Geometry: final body of the model. Coordinates: model frame, mm. A direction names the side the tool comes from. Round coordinates to 2 decimals unless told otherwise and drop trailing zeros. Loops run counter-clockwise (first coordinate to the right, second up) from the corner with the lowest first, then second, coordinate; pieces in that order, holes last. Notation, with made-up numbers: M -27,53.5 L -6,53.5 A19 cw -6,68.5 Z; hole C 38,51.5 d4. An arc over 180 degrees is marked long. Return JSON: item names as keys, results as strings.
Autodesk Inventor part; units mm, degrees
ref_plane "Start plane" through (0, 0, 0) normal (0, 0, 1) x (1, 0, 0)
ref_plane "End plane" through (0, 0, 2200) normal (0, 0, 1) x (1, 0, 0)
ref_plane "YZ Plane" through (0, 0, 0) normal (1, 0, 0) x (0, 1, 0)
ref_plane "Start plane" through (0, 0, 0) normal (0, 0, 1) x (1, 0, 0)
ref_plane "End plane" through (0, 0, 2200) normal (0, 0, 1) x (1, 0, 0)
sketch "Sketch" plane through (0, 0, 0) normal (0, 0, 1) x (1, 0, 0)
  line L0 (-1.51, 0) -> (-1.51, 50)
  line L1 (-1.51, 50) -> (48.49, 50)
  line L2 (48.49, 50) -> (48.49, 48.3694)
  line L3 (44.4604, 43.894) -> (11.5538, 40.4354)
  line L4 (4.39, 32.4792) -> (4.39, 0)
  line L5 (4.39, 0) -> (-1.51, 0) construction
  line L6 (26.44, 50) -> (26.44, 42) construction
  line L7 (48.49, 44.3175) -> (48.49, 42) construction
  line L8 (48.49, 42) -> (26.44, 42) construction
  line L9 (0, 15) -> (0, -27) construction
  line L10 (-5.539, 0) -> (16.0067, 0) construction
  line L11 (-1.51, 0) -> (-1.51, -50)
  line L12 (-1.51, -50) -> (48.49, -50)
  line L13 (48.49, -50) -> (48.49, -48.3694)
  line L14 (44.4604, -43.894) -> (11.5538, -40.4354)
  line L15 (4.39, -32.4792) -> (4.39, 0)
  arc A0 (11.5538, 40.4354) -> (4.39, 32.4792) centre (12.39, 32.4792) ccw
  arc A1 (4.39, -32.4792) -> (11.5538, -40.4354) centre (12.39, -32.4792) ccw
  arc A2 (44.4604, 43.894) -> (48.49, 48.3694) centre (43.99, 48.3694) ccw
  arc A3 (48.49, -48.3694) -> (44.4604, -43.894) centre (43.99, -48.3694) ccw
  line L16 (0, 70) -> (0, -70) construction
  line L17 (-16.5166, 0) -> (60.3266, 0) construction
  point P0 (4.39, 39.6825)
  point P1 (48.49, -44.3175)
  point P2 (4.39, -39.6825)
  point P3 (26.44, -50)
  point P4 (26.44, -42)
  dimension "d0" = 5.9
  dimension "d1" = 50
  dimension "d2" = 50
  dimension "d3" = 8
  dimension "d4" = 22.05
  dimension "d5" = 2.3175
  dimension "d23" = 8
  dimension "d24" = 4.5
  dimension "d25" = 1.51
extrude "Body" add sketch "Sketch" along normal up to surface (2200 mm away) from surface at 0
sketch "Sketch3" plane through (0, 0, 0) normal (0, 0, 1) x (1, 0, 0)
  line L0 (0, 0) -> (10, 0)
ref_plane "Work Plane3" through (0, 0, 0) normal (0, -1, 0) x (1, 0, 0)
sketch "Sketch4" plane through (0, 0, 0) normal (0, -1, 0) x (1, 0, 0)
  line L0 (-2, 0) -> (12, 0)
  line L1 (-2, 2200) -> (12, 2200)
  dimension "d29" = 2200
equation "\"d0\" = G_T"
equation "\"d1\" = 0.5 * G_H"
equation "\"d2\" = G_W"
equation "\"d3\" = G_T1"
equation "\"d4\" = G_C"
equation "\"d23\" = G_IR"
equation "\"d24\" = G_ER"
equation "\"d25\" = ex"
equation "\"d6\" = G_L"
equation "\"G_W\" = 50"
equation "\"G_T\" = 5.9"
equation "\"G_T1\" = 8"
equation "\"G_NG\" = 0.105104"
equation "\"G_ER\" = 4.5"
equation "\"G_IR\" = 8"
equation "\"G_C\" = 22.05"
equation "\"G_L\" = d29"
equation "\"ex\" = 1.51"
equation "\"G_OFFSET_START\" = 0"
equation "\"G_OFFSET_END\" = 0"
properties part number "ISO 657/11 - CH 100 x 10 - 2200" material "Steel, Mild"
Q1. Reachability of faces 1 (the flat face through (4.39, 0, 1085)), 2 (the flat face through (-1.51, 1, 1085)) from +Z, -Z, +X, -X, +Y, -Y: full face, straight path, thin tool, end or side. Return the list, or none.
Determined:
{"face 1": "+Z, -Z, +X", "face 2": "+Z, -Z, -X, +Y, -Y"}
Q2. Section query B-B (z = 761.5). Output: boundary loops of the cut face in (x, y), plus the area to 3 significant figures.
Determined:
{"outline": "M -1.51,-50 L 48.49,-50 L 48.49,-48.37 A4.5 ccw 44.46,-43.89 L 11.55,-40.44 A8 cw 4.39,-32.48 L 4.39,32.48 A8 cw 11.55,40.44 L 44.46,43.89 A4.5 ccw 48.49,48.37 L 48.49,50 L -1.51,50 Z", "area": "1,310 mm^2"}
Q3. Material intervals for L1, parallel to Y at x = 44, z = 702; L2, parallel to Y at x = 13.5, z = 538.5; L3, parallel to X at y = 33, z = 314.5, sorted ascending.
Determined:
{"L1": "y = -50 to -43.85, 43.85 to 50", "L2": "y = -50 to -40.64, 40.64 to 50", "L3": "x = -1.51 to 4.41"}
Q4. Section query C-C (y = -16). Output: boundary loops of the cut face in (x, z).
Determined:
{"outline": "M -1.51,0 L 4.39,0 L 4.39,2200 L -1.51,2200 Z"}
Q5. Section query A-A (x = 19.5). Output: boundary loops of the cut face in (y, z), plus the area to 3 significant figures.
Determined:
{"outline": "M -50,0 L -41.27,0 L -41.27,2200 L -50,2200 Z; M 41.27,0 L 50,0 L 50,2200 L 41.27,2200 Z", "area": "38,400 mm^2"}
Q6. Pin query (flat end, axial travel): pin 1 (4 mm diameter, centred on y = 10, z = 1382, fed in from +X). Return the tip coordinate at first contact, or that it passes through.
Determined:
{"pin 1": "stops at x = 4.39"}
